Autodesk Inventor part; units mm, degrees
ref_plane "YZ Plane" through (0, 0, 0) normal (1, 0, 0) x (0, 1, 0)
ref_plane "XZ Plane" through (0, 0, 0) normal (0, 1, 0) x (-1, 0, 0)
ref_plane "XY Plane" through (0, 0, 0) normal (0, 0, 1) x (1, 0, 0)
sketch "Sketch1" plane through (0, 0, 0) normal (0, 0, 1) x (1, 0, 0)
  circle A0 centre (0, 0) radius 10 construction
  circle A1 centre (0, 0) radius 11.5
  arc A2 (-3.7696, 9.8) -> (3.7696, 9.8) centre (0, 0) ccw
  line L0 (-3.7696, 9.8) -> (3.7696, 9.8)
  point P0 (0, 0)
  dimension "d0" = 23
  dimension "d1" = 21
  dimension "d2" = 9.8
extrude "Extrusion1" add sketch "Sketch1" against normal blind 10
pattern_circular "Circular Pattern1" count 3 over 360 about axis through (0, 0, 0) along (0, 0, -1) of "Extrusion1"
sketch "Sketch2" plane through (0, 0, 0) normal (0, 0, 1) x (1, 0, 0)
  circle A0 centre (0, 0) radius 11.5
  line L0 (-3.7696, 9.8) -> (3.7696, 9.8)
  arc A1 (10.3719, -1.6354) -> (3.7696, 9.8) centre (0, 0) ccw
  line L1 (10.3719, -1.6354) -> (6.6022, -8.1646)
  arc A2 (-6.6022, -8.1646) -> (6.6022, -8.1646) centre (0, 0) ccw
  line L2 (-6.6022, -8.1646) -> (-10.3719, -1.6354)
  arc A3 (-3.7696, 9.8) -> (-10.3719, -1.6354) centre (0, 0) ccw
  line L3 (-2, -1.5) -> (2, -1.5)
  line L4 (2, 1.5) -> (-2, 1.5)
  arc A4 (-2.5, 0) -> (2.5, 0) centre (0, 0) ccw construction
  line L5 (-2.0494, -1.6) -> (2.0494, -1.6)
  line L6 (-2.0494, 1.6) -> (2.0857, 1.6)
  arc A5 (2.0494, -1.6) -> (2.0494, 1.6) centre (0, 0) ccw
  arc A6 (-2.0494, 1.6) -> (-2.0494, -1.6) centre (0, 0) ccw
  point P0 (0, 0)
  dimension "d11" = 0.1
  dimension "d12" = 0.1
extrude "Extrusion2" add sketch "Sketch2" along normal blind 6 contours A0 | L0 A1 L1 A2 L2 A3
chamfer "Chamfer1" distance 4 angle 45 1 edges at (-11.5, 0, 6)
properties part number "02_WG_writer_clutch"
Source: CAD feature listing. Evaluate the final solid. Frame: model axes, mm. A direction names the side the tool comes from. Give positions to 0.01 mm unless a question says otherwise; leave off trailing zeros. Write each loop counter-clockwise with the first axis right and the second up, starting at its lowest first coordinate (ties: lowest second). Pieces come first, ordered by that corner, then holes. Notation, with made-up numbers: M 9,86.5 L 41,86.5 A15 ccw 41,106.5 Z; hole C 5,-1 d4. An arc over 180 degrees is marked long. Return JSON: item names as keys, results as strings. Group by question number.
1) Ray query, L1, parallel to Z at x = -5, y = 2.75; L2, parallel to X at y = 5.5, z = -7; L3, parallel to Y at x = -9.5, z = -8.5. Return the intervals inside material, ascending.
2) Draft query along X for faces 4 (the face through (8, -7, -10)), 5 (the face through (0, 9.8, -5)), 6 (the face through (-1.68, 7.566, 5.75)). Return one class per face: released by +X, released by -X, zero draft, split by the parting line, or undercut.
3) Set-up query: faces 1 (the face through (0, 2, 6)), 2 (the face through (2.6, 0, 3)), 3 (the face through (8.513, -4.854, -4.93)). Return all of +Z, -Z, +X, -X, +Y, -Y with unobstructed straight access to the full face (end or side cutting, diameter ignored); none if empty.
4) Cut plane B-B, the plane y = 0. Output: boundary loops of the cut face in (x, z), then the cut area to 3 significant figures.
5) Cut plane C-C, the plane x = 0. Output: boundary loops of the cut face in (y, z).
6) First-contact query: pin 1 Ø5 at (y, z) = (-3, -7.5) entering from +X; pin 2 Ø5 at (y, z) = (-4, 0) entering from -X; pin 3 Ø3.5 at (x, z) = (0, 4) entering from -Y. Flat tips, straight axial feed; report the tip coordinate or a pass-through.
7) Cut plane A-A, the plane z = -7.25. Output: boundary loops of the cut face in (x, y), then the cut area to 3 significant figures.
8) Cut plane D-D, the plane z = 4.5. Output: boundary loops of the cut face in (x, y).
Data:
{
 "1": {"L1": "z = 0 to 6", "L2": "x = -10.1 to -8.94, 8.94 to 10.1", "L3": "y = -6.48 to -3.15, 4.47 to 6.48"},
 "2": {"face 4": "zero draft", "face 5": "undercut", "face 6": "split by the parting line"},
 "3": {"face 1": "+Z, +X, -X, +Y, -Y", "face 2": "+Z, -Z", "face 3": "-Z"},
 "4": {"outline": "M -11.5,-10 L -10.5,-10 L -10.5,0 L -2.6,0 L -2.6,6 L -7.5,6 L -11.5,2 Z; M 2.6,0 L 10.5,0 L 10.5,-10 L 11.5,-10 L 11.5,2 L 7.5,6 L 2.6,6 Z", "area": "111 mm²"},
 "5": {"outline": "M -11.5,-10 L -10.5,-10 L -10.5,0 L -1.6,0 L -1.6,6 L -7.5,6 L -11.5,2 Z; M 1.6,0 L 9.8,0 L 9.8,-10 L 11.5,-10 L 11.5,2 L 7.5,6 L 1.6,6 Z"},
 "6": {"pin 1": "stops at x = 11.49", "pin 2": "stops at x = -11.4", "pin 3": "stops at y = -11.25"},
 "7": {"outline": "C 0,0 d23; hole M -10.37,-1.64 L -6.6,-8.16 A10.5 ccw 6.6,-8.16 L 10.37,-1.64 A10.5 ccw 3.77,9.8 L -3.77,9.8 A10.5 ccw Z", "area": "79.7 mm²"},
 "8": {"outline": "C 0,0 d18; hole M -2.05,-1.6 L 2.05,-1.6 A2.6 ccw 2.05,1.6 L -2.05,1.6 A2.6 ccw Z"}
}
